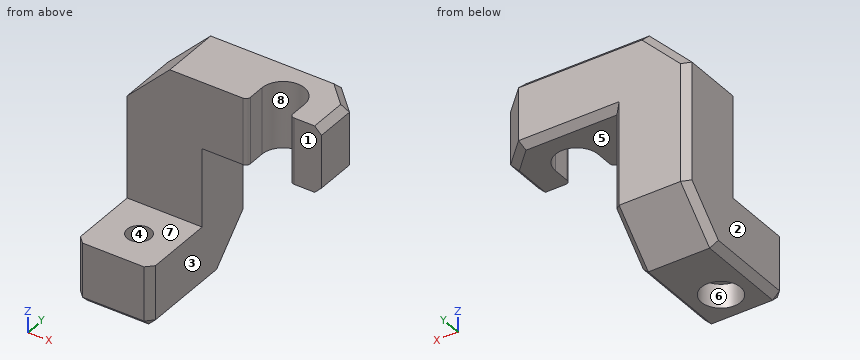
from build123d import *

# Parameters (mm, degrees)
BOSS_EXTRUDE1_DEPTH = 11.176
SKETCH2_W           = 9.906
SKETCH2_H           = 9.906
BOSS_EXTRUDE2_DEPTH = 17.78
CUT_EXTRUDE1_REACH  = 43.411
SKETCH3_R           = 3.175
CUT_EXTRUDE2_REACH  = 49.167
SKETCH4_R           = 1.778
SKETCH5_R           = 2.921
CUT_EXTRUDE3_DEPTH  = 3.556
FILLET8_R           = 0.635
CHAMFER1_SIZE       = 6.35
CHAMFER2_SIZE       = 6.35
CHAMFER3_SIZE       = 3.81
CHAMFER4_SIZE       = 1.016
CHAMFER5_SIZE       = 1.016


# Read off the part's stored shape, not the designer's step: Boss-Extrude1
with BuildPart() as part:
    # Boss-Extrude1 outline → Boss-Extrude1 (new body)
    with BuildSketch(Plane(origin=(0, 0, 0), x_dir=(0, 0, -1), z_dir=(1, 0, 0))):
        Polygon((9.099769579, 0.0001), (9.099769579, 21.082), (-21.59, 21.082), (-21.59, 11.176), (0, 11.176), (0, 0.0001), align=None)
    extrude(amount=BOSS_EXTRUDE1_DEPTH)

    # Sketch2 → Boss-Extrude2 (add)
    with BuildSketch(Plane(origin=(11.176, 0, 0), x_dir=(0, 0, -1), z_dir=(1, 0, 0))):
        with Locations((-16.637, 16.129)):
            Rectangle(SKETCH2_W, SKETCH2_H)
    extrude(amount=BOSS_EXTRUDE2_DEPTH)

    # Sketch3 → Cut-Extrude1 (cut, up to next)
    with BuildSketch(Plane(origin=(0, 0, 11.684), x_dir=(-1, 0, 0), z_dir=(0, 0, -1)), mode=Mode.PRIVATE) as cut_extrude1_sk1:
        with Locations((-21.082, 14.351)):
            Circle(SKETCH3_R)
    cut_extrude1_tool1 = extrude(cut_extrude1_sk1.sketch, amount=-CUT_EXTRUDE1_REACH, mode=Mode.PRIVATE) & part.part
    # Sketch3 → Cut-Extrude1 (cut, up to next)
    with BuildSketch(Plane(origin=(0, 0, 11.684), x_dir=(-1, 0, 0), z_dir=(0, 0, -1)), mode=Mode.PRIVATE) as cut_extrude1_sk2:
        with BuildLine():
            ThreePointArc((-21.082, 11.176), (-23.32706403, 12.10593597), (-24.257, 14.351))
            Line((-24.257, 14.351), (-24.257, 11.176))
            Line((-24.257, 11.176), (-21.082, 11.176))
        make_face()
    cut_extrude1_tool2 = extrude(cut_extrude1_sk2.sketch, amount=-CUT_EXTRUDE1_REACH, mode=Mode.PRIVATE) & part.part
    # Sketch3 → Cut-Extrude1 (cut, up to next)
    with BuildSketch(Plane(origin=(0, 0, 11.684), x_dir=(-1, 0, 0), z_dir=(0, 0, -1)), mode=Mode.PRIVATE) as cut_extrude1_sk3:
        with BuildLine():
            Line((-17.907, 11.176), (-17.907, 14.351))
            ThreePointArc((-17.907, 14.351), (-18.83693597, 12.10593597), (-21.082, 11.176))
            Line((-21.082, 11.176), (-17.907, 11.176))
        make_face()
    cut_extrude1_tool3 = extrude(cut_extrude1_sk3.sketch, amount=-CUT_EXTRUDE1_REACH, mode=Mode.PRIVATE) & part.part
    add(cut_extrude1_tool1.solids().sort_by_distance((21.082, 14.351, 11.684))[0], mode=Mode.SUBTRACT)
    add(cut_extrude1_tool2.solids().sort_by_distance((23.547807, 11.885193, 11.684))[0], mode=Mode.SUBTRACT)
    add(cut_extrude1_tool3.solids().sort_by_distance((18.616193, 11.885193, 11.684))[0], mode=Mode.SUBTRACT)

    # Sketch4 → Cut-Extrude2 (cut, up to next)
    with BuildSketch(Plane(origin=(0, 0, -9.099769579), x_dir=(-1, 0, 0), z_dir=(0, 0, -1)), mode=Mode.PRIVATE) as cut_extrude2_sk1:
        with Locations((-5.588, 5.5881)):
            Circle(SKETCH4_R)
    cut_extrude2_tool1 = extrude(cut_extrude2_sk1.sketch, amount=-CUT_EXTRUDE2_REACH, mode=Mode.PRIVATE) & part.part
    add(cut_extrude2_tool1.solids().sort_by_distance((5.588, 5.5881, -9.09977))[0], mode=Mode.SUBTRACT)

    # Sketch5 → Cut-Extrude3 (cut)
    with BuildSketch(Plane(origin=(0, 0, -9.099769579), x_dir=(-1, 0, 0), z_dir=(0, 0, -1))):
        with Locations((-5.588, 5.5881)):
            Circle(SKETCH5_R)
    extrude(amount=-CUT_EXTRUDE3_DEPTH, mode=Mode.SUBTRACT)

    # Fillet8
    fillet8_edges = [part.edges().sort_by_distance(p)[0] for p in [
        (24.257, 11.176, 16.637),
        (17.907, 11.176, 16.637),
    ]]
    fillet(fillet8_edges, radius=FILLET8_R)

    # Chamfer1
    chamfer1_edges = [part.edges().sort_by_distance(p)[0] for p in [
        (5.588, 21.082, -9.099769579),
    ]]
    chamfer(chamfer1_edges, length=CHAMFER1_SIZE)

    # Chamfer2
    chamfer2_edges = [part.edges().sort_by_distance(p)[0] for p in [
        (0, 16.129, 21.59),
    ]]
    chamfer(chamfer2_edges, length=CHAMFER2_SIZE)

    # Chamfer3
    chamfer3_edges = [part.edges().sort_by_distance(p)[0] for p in [
        (28.956, 21.082, 16.637),
    ]]
    chamfer(chamfer3_edges, length=CHAMFER3_SIZE)

    # Chamfer4
    chamfer4_edges = [part.edges().sort_by_distance(p)[0] for p in [
        (28.956, 14.224, 21.59),
        (27.051, 19.177, 21.59),
        (15.748, 21.082, 21.59),
        (28.956, 14.224, 11.684),
        (27.051, 19.177, 11.684),
        (18.161, 21.082, 11.684),
        (11.176, 21.082, 4.46711521),
        (11.176, 17.907, -5.924769579),
        (0, 21.082, 6.24511521),
        (0, 17.907, -5.924769579),
        (0, 7.36605, -9.099769579),
        (11.176, 7.36605, -9.099769579),
        (0, 0.0001, -4.54988479),
        (5.588, 0.0001, -9.099769579),
        (11.176, 0.0001, -4.54988479),
    ]]
    chamfer(chamfer4_edges, length=CHAMFER4_SIZE)

    # Chamfer5
    chamfer5_edges = [part.edges().sort_by_distance(p)[0] for p in [
        (3.175, 21.082, 18.415),
    ]]
    chamfer(chamfer5_edges, length=CHAMFER5_SIZE)


solid = part.part
Verification items for the finished model (mm, model axes). Face numbers are marked on the shaded views. A direction names the side the tool comes from. Coordinates: 2 decimals unless noted, no trailing zeros. Order: outer loops, then holes, each group sorted by start corner. A loop starts at its lowest first (then second) coordinate and runs counter-clockwise, first axis right, second up.
1. Scan lines: line 1 (Z direction, x = 5.25, y = 9); line 2 (X direction, y = 17.5, z = -3); line 3 (X direction, y = 13.25, z = 15.5). Record each from-to range of solid material in increasing order.
Results found:
line 1: z = -9.1 to 0
line 2: x = 0 to 11.18
line 3: x = 0.26 to 17.91, 24.26 to 28.96
2. Sectioned sample at C-C, the plane x = 9. Record the cut outline in (y, z).
Results found:
outline: (0, -8.08) - (1.02, -9.1) - (14.73, -9.1) - (21.08, -2.75) - (21.08, 20.57) - (20.07, 21.59) - (11.18, 21.59) - (11.18, 0) - (0, 0) - close
3. Release check for a two-part mould opening along X. For the marked faces 1, 2, 3 and 4 record: +X half, -X half, draft (parallel to the pull), parting line (faces both ways), or undercut.
Results found:
face 1: draft
face 2: -X half
face 3: +X half
face 4: undercut
4. Sectioned sample at B-B, the plane z = -1.5. Record the cut outline in (x, y).
Results found:
outline: (0, 1.02) - (1.02, 0) - (10.16, 0) - (11.18, 1.02) - (11.18, 20.07) - (10.16, 21.08) - (1.02, 21.08) - (0, 20.07) - close; hole circle Ø3.56 at (5.59, 5.59)
5. Sectioned sample at D-D, the plane z = 17.5. Record the cut outline in (x, y) (3 decimals).
Results found:
outline: (2.26, 11.176) - (17.272, 11.176) arc R0.635 ccw to (17.907, 11.811) - (17.907, 14.351) arc R3.175 cw to (24.257, 14.351) - (24.257, 11.811) arc R0.635 ccw to (24.892, 11.176) - (28.956, 11.176) - (28.956, 17.272) - (25.146, 21.082) - (3.697, 21.082) - (2.26, 20.066) - close
6. Go/stop test with flat-tipped pins: pin 1 Ø6 at (y, z) = (16, 3.5) entering from +X; pin 2 Ø10 at (x, z) = (25.5, 10.5) entering from -Y; pin 3 Ø10 at (x, y) = (23.5, 13.5) entering from -Z; pin 4 Ø12 at (x, z) = (17.5, 0) entering from -Y. Record where each tip stops, or that it passes through.
Results found:
pin 1: stops at x = 11.18
pin 2: stops at y = 11.18
pin 3: stops at z = 11.68
pin 4: passes through
7. Sectioned sample at A-A, the plane y = 6.25. Record the cut outline in (x, z).
Results found:
outline: (0, -8.08) - (1.02, -9.1) - (2.74, -9.1) - (2.74, -5.54) - (3.94, -5.54) - (3.94, 0) - (0, 0) - close; (7.24, -5.54) - (8.43, -5.54) - (8.43, -9.1) - (10.16, -9.1) - (11.18, -8.08) - (11.18, 0) - (7.24, 0) - close
8. Set-up check for the marked faces 5, 6, 7 and 8: record each of +Z, -Z, +X, -X, +Y, -Y from which the full face is reachable in a straight line by a thin tool's end or side.
Results found:
face 5: -Z, +X, +Y, -Y
face 6: -Z
face 7: +Z, +X, -X, -Y
face 8: +Z, -Z, -Y
